CAD build for the part. Positions are in the model's coordinates, mm. Give positions to 0.01 mm unless a question says otherwise; leave off trailing zeros. Order: outer loops, then holes, each group sorted by start corner. A loop starts at its lowest first (then second) coordinate and runs counter-clockwise, first axis right, second up. Notation, with made-up numbers: M -14,52.5 L 4,52.5 A4 cw 4,56.5 Z; hole C -1.5,-29 d5. An arc over 180 degrees is marked long. Put each result on its own line as item: value. Start each with the question number.
1) Cut at B-B (y = -201). Write the cut outline in (x, z), and give its area (4 significant figures).
2) Cut at A-A (x = -57). Write the cut outline in (y, z).
3) Cut at D-D (y = 129.5). Write the cut outline in (x, z), and give its area (3 significant figures).
4) Cut at C-C (x = 35). Write the cut outline in (y, z).
5) Pin check, flat tip, straight feed: pin 1 (9 mm diameter, centred on x = -57, y = -263.72, fed in from +Z). Stop position of the tip, or through.
6) Drill centre lines: line 1 (Y direction, x = 22.5, z = 7.25); line 2 (Y direction, x = -57, z = 4); line 3 (X direction, y = -242.5, z = 9.5). Where is each one in solid material? Low to high. Write a range as [from, to].
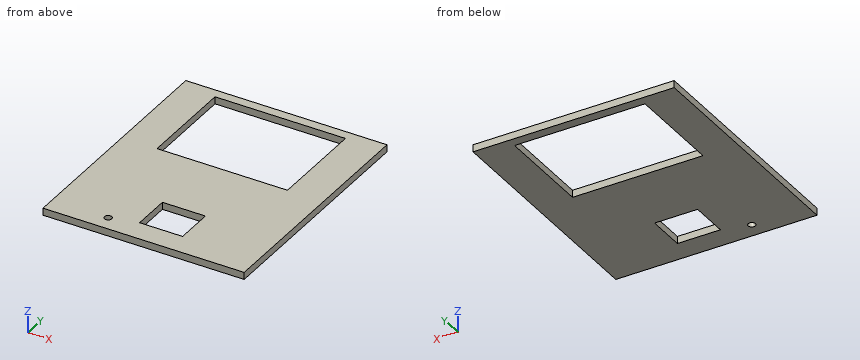
```python
from build123d import *

# Parameters (mm, degrees)
F0_W     = 421
F0_H     = 500
F0_R     = 7.5
F0_W_2   = 90
F0_H_2   = 80
F0_W_3   = 273
F0_H_3   = 203
F1_DEPTH = 15


with BuildPart() as f1:
    # F0 (on Top) → F1 (new body)
    with BuildSketch(Plane.XY):
        with Locations((36.5, -46.220626)):
            Rectangle(F0_W, F0_H)
        with Locations((-57, -263.720626)):
            Circle(F0_R, mode=Mode.SUBTRACT)
        with Locations((45, -209.220626)):
            Rectangle(F0_W_2, F0_H_2, mode=Mode.SUBTRACT)
        with Locations((35.5, 82.279374)):
            Rectangle(F0_W_3, F0_H_3, mode=Mode.SUBTRACT)
    extrude(amount=F1_DEPTH)


solid = f1.part
```
Solution:
1. outline: M -174,0 L 0,0 L 0,15 L -174,15 Z; M 90,0 L 247,0 L 247,15 L 90,15 Z
1. area: 4,965 mm²
2. outline: M -296.22,0 L -271.22,0 L -271.22,15 L -296.22,15 Z; M -256.22,0 L -19.22,0 L -19.22,15 L -256.22,15 Z; M 183.78,0 L 203.78,0 L 203.78,15 L 183.78,15 Z
3. outline: M -174,0 L -101,0 L -101,15 L -174,15 Z; M 172,0 L 247,0 L 247,15 L 172,15 Z
3. area: 2,220 mm²
4. outline: M -296.22,0 L -249.22,0 L -249.22,15 L -296.22,15 Z; M -169.22,0 L -19.22,0 L -19.22,15 L -169.22,15 Z; M 183.78,0 L 203.78,0 L 203.78,15 L 183.78,15 Z
5. pin 1: through
6. line 1: [-296.22, -249.22], [-169.22, -19.22], [183.78, 203.78]
6. line 2: [-296.22, -271.22], [-256.22, -19.22], [183.78, 203.78]
6. line 3: [-174, 0], [90, 247]
